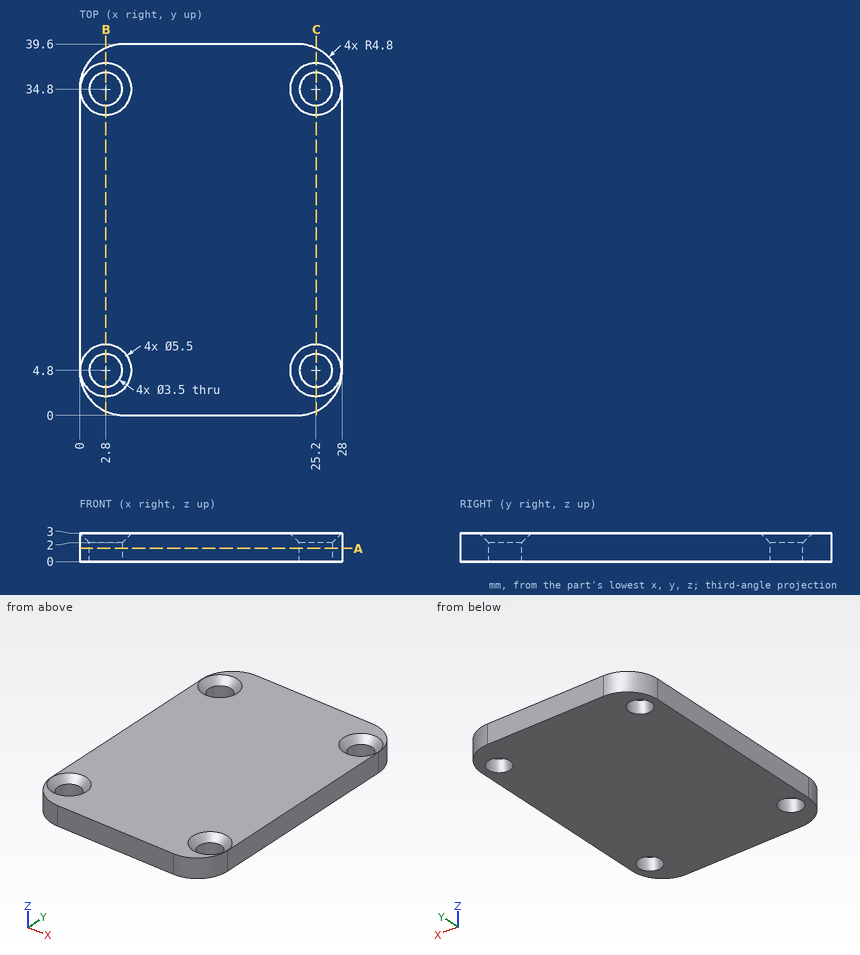
Design review of the part shown in the three views and the two pictorial views. Dimensions are in mm from the part's minimum x, y and z. Give positions to 0.01 mm unless a question says otherwise; leave off trailing zeros. Write each loop counter-clockwise with the first axis right and the second up, starting at its lowest first coordinate (ties: lowest second). Pieces come first, ordered by that corner, then holes. Notation, with made-up numbers: M -36.75,84 L -24.75,84 A9 cw -24.75,88 Z; hole C 30.5,-1.75 d11. An arc over 180 degrees is marked long. Return JSON: item names as keys, results as strings. Group by question number.
Item 1: Take a section at B-B (x = 2.8). Give the boundary of the cut face in (y, z).
Item 2: Clearance check with flat-ended pins moving along their axes: pin 1 Ø1 at (y, z) = (30, 1) entering from -X; pin 2 Ø4 at (x, y) = (25.2, 34.8) entering from +Z. State where each tip first meets the part, or that it passes through.
Item 3: Take a section at A-A (z = 1.4). Give the boundary of the cut face in (x, y).
Item 4: Take a section at C-C (x = 25.25). Count the separate pieces of the cut face and the enclosed holes in it, plus the area to 3 significant figures.
Item 5: Wall thickness on line 1 along X through (y, z) = (6.5, 2.45); line 2 along Y through (x, z) = (26, 0.35); line 3 along X through (y, z) = (36, 1.85): over which ranges is each line inside the solid? List them lowest first.
Return value:
{
 "1": {"outline": "M 0.44,0 L 3.05,0 L 3.05,2 L 2.05,3 L 0.44,3 Z; M 6.55,0 L 33.05,0 L 33.05,2 L 32.05,3 L 7.55,3 L 6.55,2 Z; M 36.55,0 L 39.16,0 L 39.16,3 L 37.55,3 L 36.55,2 Z"},
 "2": {"pin 1": "stops at x = 0", "pin 2": "stops at z = 2.25"},
 "3": {"outline": "M 0,4.8 A4.8 ccw 4.8,0 L 23.2,0 A4.8 ccw 28,4.8 L 28,34.8 A4.8 ccw 23.2,39.6 L 4.8,39.6 A4.8 ccw 0,34.8 Z; hole C 2.8,4.8 d3.5; hole C 2.8,34.8 d3.5; hole C 25.2,4.8 d3.5; hole C 25.2,34.8 d3.5"},
 "4": {"separate pieces": "3", "enclosed holes": "0", "area": "93.0 mm2"},
 "5": {"line 1": "x = 0 to 1.4, 4.2 to 23.8, 26.6 to 28", "line 2": "y = 0.9 to 3.24, 6.36 to 33.24, 36.36 to 38.7", "line 3": "x = 0.15 to 1.53, 4.07 to 23.93, 26.47 to 27.85"}
}
